Can you work these out from the drawing? Everything is in mm from the part's minimum corner. A direction names the side the tool comes from. Give positions to 0.01 mm unless a question says otherwise; leave off trailing zeros. Loops run counter-clockwise (first coordinate to the right, second up) from the corner with the lowest first, then second, coordinate; pieces in that order, holes last.
Q1. If we section it at B-B (y = 7.75): Please give me the cut outline in (x, z).
Q2. If we section it at D-D (y = 4.5): Please give me the cut outline in (x, z).
Q3. If we section it at C-C (x = 61): Please give me the cut outline in (y, z).
Q4. For the marked faces 1 and 2, which set-ups out of +Z, -Z, +X, -X, +Y, -Y let a thin tool reach every point of the face, with its end or its side?
Q5. I need wall thicknesses on line 1 (Y direction, x = 34, z = 1); line 2 (Y direction, x = 50, z = 7.5); line 3 (Z direction, x = 8, y = 3.75). Which ranges of each line are inside material? Lowest first, please.
Q6. Will these pins go through, and if not, where does the flat tip stop? P1, Ø6, axis at y = 2.5, z = 7, coming from the +X side; P2, Ø1.5, axis at x = 48, y = 3, coming from the +Z side; P3, Ø8.5, axis at x = 21, z = 19.5, coming from the -Y side.
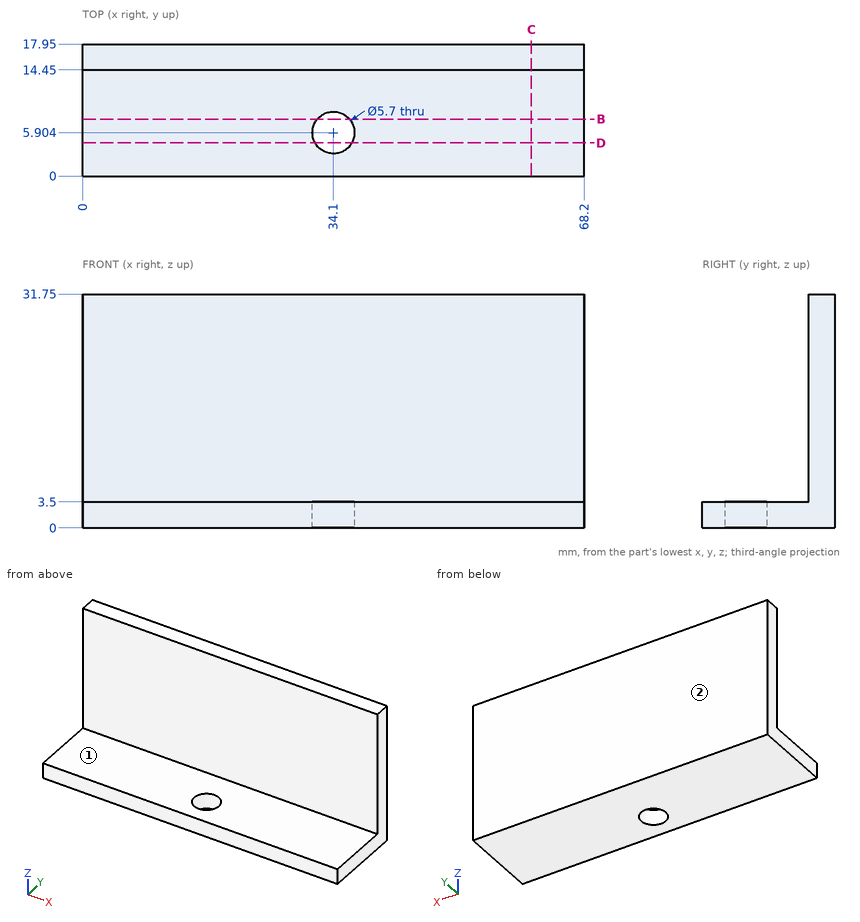
Check sheet entries:
1. outline: (0, 0) - (31.93, 0) - (31.93, 3.5) - (0, 3.5) - close; (36.27, 0) - (68.2, 0) - (68.2, 3.5) - (36.27, 3.5) - close
2. outline: (0, 0) - (31.62, 0) - (31.62, 3.5) - (0, 3.5) - close; (36.58, 0) - (68.2, 0) - (68.2, 3.5) - (36.58, 3.5) - close
3. outline: (0, 0) - (17.95, 0) - (17.95, 31.75) - (14.45, 31.75) - (14.45, 3.5) - (0, 3.5) - close
4. face 1: +Z, +X, -X, -Y
4. face 2: +Z, -Z, +X, -X, +Y
5. line 1: y = 0 to 3.06, 8.75 to 17.95
5. line 2: y = 14.45 to 17.95
5. line 3: z = 0 to 3.5
6. P1: passes through
6. P2: stops at z = 3.5
6. P3: stops at y = 14.45
